Read the model definition and answer for the solid it produces. Units are mm, in the model's axes. A direction names the side the tool comes from. Coordinates: 2 decimals unless noted, no trailing zeros. Loops run counter-clockwise (first coordinate to the right, second up) from the corner with the lowest first, then second, coordinate; pieces in that order, holes last. Notation, with made-up numbers: (0.5, 63) -> (52.5, 63) arc R24 ccw to (52.5, 74) -> close; hole circle Ø10 at (35, 1). An arc over 180 degrees is marked (long way). Answer as a JSON object with one key per item and string values. Group by question number.
1) Section C-C, the plane x = -10.5 is taken. Give the vertices of the cut face in (y, z), plus the area to 3 significant figures.
2) Section D-D, the plane z = 1.2 is taken. Give the vertices of the cut face in (x, y), plus the area to 3 significant figures.
3) Determine the mould class of faces 1 (the face through (9, -9, 5)), 2 (the face through (-1.11, 17.51, 2.21)), 3 (the face through (-4.336, -19.524, 2.212)) for opening direction Y: released by +Y, released by -Y, zero draft, split by the parting line, or undercut.
4) Flat-ended cylindrical pins translate along their axes: P1, Ø1, axis at y = 13, z = 1, coming from the +X side; P2, Ø3, axis at x = -7.5, z = 0.5, coming from the +Y side; P3, Ø2, axis at x = 1, z = 3, coming from the +Y side. Find the tip coordinate at first contact, or state that the pin passes through.
5) Which of the six approach directions +Z, -Z, +X, -X, +Y, -Y give full straight-line access (tool end or side, diameter ignored) to faces 4 (the face through (-0.54, -18.94, 2.21)), 5 (the face through (-11.99, 0.53, 2.46))?
6) Section B-B, the plane y = 16.5 is taken. Give the vertices of the cut face in (x, z).
7) Consider probe 1 along Y at (x, z) = (0, 0.75); probe 2 along Y at (x, z) = (0, -0.05); probe 3 along X at (y, z) = (10, 3.65). Determine where each line is inside the solid, lowest interval first. Write a range as [from, to].
8) Section A-A, the plane x = 0 is taken. Give the vertices of the cut face in (y, z).
from build123d import *

# Parameters (mm, degrees)
SKETCH1_R           = 20
SKETCH1_R_2         = 2.5
SKETCH1_R_3         = 1.5
SKETCH1_R_4         = 12
BOSS_EXTRUDE1_DEPTH = 5
BOSS_EXTRUDE2_START = -0.5
SKETCH1_3_R         = 20
SKETCH1_3_R_2       = 2.5
SKETCH1_3_R_3       = 1.5
SKETCH1_3_R_4       = 12
SKETCH1_3_R_5       = 11
BOSS_EXTRUDE2_DEPTH = 0.5


with BuildPart() as part:
    # Sketch1 → Boss-Extrude1 (new body)
    with BuildSketch(Plane.XY):
        Circle(SKETCH1_R)
        with Locations((14.289419162, 8.25)):
            Circle(SKETCH1_R_2, mode=Mode.SUBTRACT)
        with Locations((-14.289419162, 8.25)):
            Circle(SKETCH1_R_2, mode=Mode.SUBTRACT)
        with Locations((0, -16.5)):
            Circle(SKETCH1_R_2, mode=Mode.SUBTRACT)
        with Locations((-14.289419162, -8.25)):
            Circle(SKETCH1_R_3, mode=Mode.SUBTRACT)
        with Locations((14.289419162, -8.25)):
            Circle(SKETCH1_R_3, mode=Mode.SUBTRACT)
        with Locations((0, 16.5)):
            Circle(SKETCH1_R_3, mode=Mode.SUBTRACT)
        Circle(SKETCH1_R_4, mode=Mode.SUBTRACT)
    extrude(amount=BOSS_EXTRUDE1_DEPTH)

    # Sketch1_3 → Boss-Extrude2 (add)
    # profile 1 of 2: a face of its own
    with BuildSketch(Plane.XY.offset(BOSS_EXTRUDE2_START)):
        Circle(SKETCH1_3_R)
        with Locations((14.289419162, 8.25)):
            Circle(SKETCH1_3_R_2, mode=Mode.SUBTRACT)
        with Locations((-14.289419162, 8.25)):
            Circle(SKETCH1_3_R_2, mode=Mode.SUBTRACT)
        with Locations((0, -16.5)):
            Circle(SKETCH1_3_R_2, mode=Mode.SUBTRACT)
        with Locations((-14.289419162, -8.25)):
            Circle(SKETCH1_3_R_3, mode=Mode.SUBTRACT)
        with Locations((14.289419162, -8.25)):
            Circle(SKETCH1_3_R_3, mode=Mode.SUBTRACT)
        with Locations((0, 16.5)):
            Circle(SKETCH1_3_R_3, mode=Mode.SUBTRACT)
        Circle(SKETCH1_3_R_4, mode=Mode.SUBTRACT)
    # profile 2 of 2: a face of its own
    with BuildSketch(Plane.XY.offset(BOSS_EXTRUDE2_START)):
        Circle(SKETCH1_3_R_4)
        Circle(SKETCH1_3_R_5, mode=Mode.SUBTRACT)
    extrude(amount=BOSS_EXTRUDE2_DEPTH)


solid = part.part
Determined:
{
 "1": {"outline": "(-17.02, -0.5) -> (-3.28, -0.5) -> (-3.28, 0) -> (-5.81, 0) -> (-5.81, 5) -> (-17.02, 5) -> close; (3.28, -0.5) -> (17.02, -0.5) -> (17.02, 5) -> (5.81, 5) -> (5.81, 0) -> (3.28, 0) -> close", "area": "126 mm²"},
 "2": {"outline": "circle Ø40 at (0, 0); hole circle Ø5 at (-14.29, 8.25); hole circle Ø3 at (-14.29, -8.25); hole circle Ø24 at (0, 0); hole circle Ø5 at (0, -16.5); hole circle Ø3 at (0, 16.5); hole circle Ø5 at (14.29, 8.25); hole circle Ø3 at (14.29, -8.25)", "area": "724 mm²"},
 "3": {"face 1": "zero draft", "face 2": "undercut", "face 3": "split by the parting line"},
 "4": {"P1": "x = 15.61", "P2": "y = 19.08", "P3": "y = 20"},
 "5": {"face 4": "+Z, -Z", "face 5": "+Z"},
 "6": {"outline": "(-11.3, -0.5) -> (-1.5, -0.5) -> (-1.5, 5) -> (-11.3, 5) -> close; (1.5, -0.5) -> (11.3, -0.5) -> (11.3, 5) -> (1.5, 5) -> close"},
 "7": {"probe 1": "[-20, -19], [-14, -12], [12, 15], [18, 20]", "probe 2": "[-20, -19], [-14, -11], [11, 15], [18, 20]", "probe 3": "[-17.32, -16.07], [-12.5, -6.63], [6.63, 12.5], [16.07, 17.32]"},
 "8": {"outline": "(-20, -0.5) -> (-19, -0.5) -> (-19, 5) -> (-20, 5) -> close; (-14, -0.5) -> (-11, -0.5) -> (-11, 0) -> (-12, 0) -> (-12, 5) -> (-14, 5) -> close; (11, -0.5) -> (15, -0.5) -> (15, 5) -> (12, 5) -> (12, 0) -> (11, 0) -> close; (18, -0.5) -> (20, -0.5) -> (20, 5) -> (18, 5) -> close"}
}
